```python
from build123d import *

# Parameters (mm, degrees)
SKETCH_1_W                     = 80
SKETCH_1_H                     = 60
EXTRUDE_1_DEPTH                = 8
HOLE_WIZARD_M3_5_1_D           = 4
HOLE_WIZARD_M3_5_1_CBORE_D     = 8
HOLE_WIZARD_M3_5_1_CBORE_DEPTH = 2
SKETCH_14_W                    = 80
SKETCH_14_H                    = 2
SKETCH_14_W_2                  = 2
SKETCH_14_H_2                  = 16
CUT_EXTRUDE_1_DEPTH            = 1
CUT_EXTRUDE_2_REACH            = 92.174
SKETCH_15_R                    = 4.75
SKETCH_17_R                    = 11.5
CUT_EXTRUDE_4_DEPTH            = 4
SKETCH_18_R                    = 6
CUT_EXTRUDE_5_DEPTH            = 3
CHAMFER_1_SIZE                 = 1.499999999
CHAMFER_1_SIZE2                = 1.500000001
CHAMFER_2_SIZE                 = 1
SKETCH_20_W                    = 80
SKETCH_20_H                    = 6
CUT_EXTRUDE_6_DEPTH            = 1
SKETCH_21_W                    = 80
SKETCH_21_H                    = 4
CUT_EXTRUDE_7_DEPTH            = 1
SKETCH_22_W                    = 80
SKETCH_22_H                    = 2
CUT_EXTRUDE_8_DEPTH            = 1
SKETCH_23_R                    = 1
CUT_EXTRUDE_9_DEPTH            = 1
CUT_EXTRUDE_10_REACH           = 92.174
SKETCH_24_W                    = 80
SKETCH_24_H                    = 10


with BuildPart() as part:
    # 草图1 → 凸台-拉伸1 (new body)
    with BuildSketch(Plane.XY.offset(8)):
        with Locations((40, 10.833333333)):
            Rectangle(SKETCH_1_W, SKETCH_1_H)
    extrude(amount=-EXTRUDE_1_DEPTH)

    # M3.5 六角头机械螺钉的柱形沉头孔1 (through all)
    with Locations(Plane.XY.offset(8)):
        with Locations((8, 10.833333333), (72, 10.833333333)):
            CounterBoreHole(HOLE_WIZARD_M3_5_1_D / 2, HOLE_WIZARD_M3_5_1_CBORE_D / 2, HOLE_WIZARD_M3_5_1_CBORE_DEPTH)

    # 草图14 → 切除-拉伸1 (cut)
    with BuildSketch(Plane.XY.offset(8)):
        with Locations((40, 37.833333333)):
            Rectangle(SKETCH_14_W, SKETCH_14_H)
        Polygon((15, 40.833333333), (31, 24.833333333), (32.414213562, 26.247546896), (16.414213562, 42.247546896), align=None)
        with Locations((7, 32.833333333)):
            Rectangle(SKETCH_14_W_2, SKETCH_14_H_2)
        with Locations((40, 32.833333333)):
            Rectangle(SKETCH_14_W_2, SKETCH_14_H_2)
        with Locations((73, 32.833333333)):
            Rectangle(SKETCH_14_W_2, SKETCH_14_H_2)
        Polygon((47.585786438, 26.247546896), (63.585786438, 42.247546896), (65, 40.833333333), (49, 24.833333333), align=None)
    extrude(amount=-CUT_EXTRUDE_1_DEPTH, mode=Mode.SUBTRACT)

    # 草图15 → 切除-拉伸2 (cut, up to next)
    with BuildSketch(Plane.XY.offset(8), mode=Mode.PRIVATE) as cut_extrude_2_sk1:
        with Locations((40, 10.833333333)):
            Circle(SKETCH_15_R)
    cut_extrude_2_tool1 = extrude(cut_extrude_2_sk1.sketch, amount=-CUT_EXTRUDE_2_REACH, mode=Mode.PRIVATE) & part.part
    add(cut_extrude_2_tool1.solids().sort_by_distance((40, 10.833333, 8))[0], mode=Mode.SUBTRACT)

    # 草图17 → 切除-拉伸4 (cut)
    with BuildSketch(Plane.XY.offset(8)):
        with Locations((40, 10.833333333)):
            Circle(SKETCH_17_R)
    extrude(amount=-CUT_EXTRUDE_4_DEPTH, mode=Mode.SUBTRACT)

    # 草图18 → 切除-拉伸5 (cut)
    with BuildSketch(Plane(origin=(0, 0, 0), x_dir=(-1, 0, 0), z_dir=(0, 0, -1))):
        with Locations((-40, 10.833333333)):
            Circle(SKETCH_18_R)
    extrude(amount=-CUT_EXTRUDE_5_DEPTH, mode=Mode.SUBTRACT)

    # 倒角1
    chamfer_1_edges = [part.edges().sort_by_distance(p)[0] for p in [
        (74, 10.833333333, 0),
        (10, 10.833333333, 0),
    ]]
    chamfer_1_side = [part.faces().sort_by_distance(p)[0] for p in [
        (79, 10.833333333, 0),
    ]]
    chamfer(chamfer_1_edges, length=CHAMFER_1_SIZE, length2=CHAMFER_1_SIZE2, reference=chamfer_1_side[0])

    # 倒角2
    chamfer_2_edges = [part.edges().sort_by_distance(p)[0] for p in [
        (40, 40.833333333, 0),
    ]]
    chamfer(chamfer_2_edges, length=CHAMFER_2_SIZE)

    # 草图20 → 切除-拉伸6 (cut)
    with BuildSketch(Plane.XY.offset(8)):
        with Locations((40, -16.166666667)):
            Rectangle(SKETCH_20_W, SKETCH_20_H)
    extrude(amount=-CUT_EXTRUDE_6_DEPTH, mode=Mode.SUBTRACT)

    # 草图21 → 切除-拉伸7 (cut)
    with BuildSketch(Plane.XY.offset(7)):
        with Locations((40, -17.166666667)):
            Rectangle(SKETCH_21_W, SKETCH_21_H)
    extrude(amount=-CUT_EXTRUDE_7_DEPTH, mode=Mode.SUBTRACT)

    # 草图22 → 切除-拉伸8 (cut)
    with BuildSketch(Plane.XY.offset(6)):
        with Locations((40, -18.166666667)):
            Rectangle(SKETCH_22_W, SKETCH_22_H)
    extrude(amount=-CUT_EXTRUDE_8_DEPTH, mode=Mode.SUBTRACT)

    # 草图23 → 切除-拉伸9 (cut)
    with BuildSketch(Plane.XY.offset(8)):
        with Locations((7, 24.833333333)):
            Circle(SKETCH_23_R)
        with Locations((31.707106781, 25.540440115)):
            Circle(SKETCH_23_R)
        with Locations((40, 24.833333333)):
            Circle(SKETCH_23_R)
        with Locations((48.292893219, 25.540440115)):
            Circle(SKETCH_23_R)
        with Locations((73, 24.833333333)):
            Circle(SKETCH_23_R)
    extrude(amount=-CUT_EXTRUDE_9_DEPTH, mode=Mode.SUBTRACT)

    # 草图24 → 切除-拉伸10 (cut, up to next)
    with BuildSketch(Plane.XY.offset(8), mode=Mode.PRIVATE) as cut_extrude_10_sk1:
        with Locations((40, -14.166666667)):
            Rectangle(SKETCH_24_W, SKETCH_24_H)
    cut_extrude_10_tool1 = extrude(cut_extrude_10_sk1.sketch, amount=-CUT_EXTRUDE_10_REACH, mode=Mode.PRIVATE) & part.part
    add(cut_extrude_10_tool1.solids().sort_by_distance((40, -14.166667, 8))[0], mode=Mode.SUBTRACT)


solid = part.part
```
CAD build for the part. Positions are in the model's coordinates, mm. A direction names the side the tool comes from. Coordinates: 2 decimals unless noted, no trailing zeros. Order: outer loops, then holes, each group sorted by start corner. A loop starts at its lowest first (then second) coordinate and runs counter-clockwise, first axis right, second up. Notation, with made-up numbers: (78.25, -17.75) - (134.25, -17.75) arc R19 cw to (134.25, -12.75) - close; hole circle Ø6 at (37, 81.25). An arc over 180 degrees is marked (long way). Use a Markdown table: item, result. Add a question column.
(1) Pull direction X, two halves, no side cores. Call faces 5 (the face through (28.51, 11.34, 6.03)), 6 (the face through (12, 40, 8)), 7 (the face through (0, 15, 4)): +X half, -X half, draft (parallel to the pull), parting line (faces both ways), or undercut.
(2) Flat gauge pins, fed straight in: pin 1 (1.1 mm diameter, centred on y = 40, z = 7.5, fed in from -X); pin 2 (3.5 mm diameter, centred on x = 37, y = 12.5, fed in from -Z); pin 3 (5 mm diameter, centred on x = 8, y = 10.83, fed in from -Z). Where does each tip first touch, or does it go through?
(3) Drill centre lines: line 1 along Y through (x, z) = (40, 5.35); line 2 along X through (y, z) = (9.5, 2.75); line 3 along Y through (x, z) = (40, 1.9). Where is each one in solid material? Low to high. Write a range as [from, to].
(4) Saw through at B-B (y = 19). Give the cut face in (x, z).
(5) Saw through at A-A (x = 40). Give the cut face in (y, z), then the cut area to 3 significant figures.
(6) Which spindle directions (+Z, -Z, +X, -X, +Y, -Y) get a long thin tool onto all of the face, cutting with end or side? Do faces 1 (the face through (70, 10, 6)), 2 (the face through (36, 8, 3)), 3 (the face through (64.014, 39.847, 7.507)), 4 (the face through (31, 19, 8)). Say none if no direction does.
Solved:
| question | item | result |
|---|---|---|
| 1 | face 5 | undercut |
| 1 | face 6 | draft |
| 1 | face 7 | -X half |
| 2 | pin 1 | stops at x = 0 |
| 2 | pin 2 | stops at z = 3 |
| 2 | pin 3 | stops at z = 1 |
| 3 | line 1 | y = [-9.17, -0.67], [22.33, 40.83] |
| 3 | line 2 | x = [0, 6.51], [9.49, 34.15], [45.85, 70.51], [73.49, 80] |
| 3 | line 3 | y = [-9.17, 4.83], [16.83, 40.83] |
| 4 | outline | (0, 0) - (80, 0) - (80, 8) - (48.1, 8) - (48.1, 4) - (31.9, 4) - (31.9, 8) - (0, 8) - close |
| 5 | outline | (-9.17, 0) - (4.83, 0) - (4.83, 3) - (6.08, 3) - (6.08, 4) - (-0.67, 4) - (-0.67, 8) - (-9.17, 8) - close; (15.58, 3) - (16.83, 3) - (16.83, 0) - (39.83, 0) - (40.83, 1) - (40.83, 7) - (23.83, 7) - (23.83, 8) - (22.33, 8) - (22.33, 4) - (15.58, 4) - close |
| 5 | area | 245 mm² |
| 6 | face 1 | +Z |
| 6 | face 2 | -Z |
| 6 | face 3 | +Z, +Y |
| 6 | face 4 | +Z, +X, -X, +Y, -Y |
